Could you check a few things on this model? Use its own coordinates, in mm. A direction names the side the tool comes from. Coordinates: 2 decimals unless noted, no trailing zeros. Loops run counter-clockwise (first coordinate to the right, second up) from the corner with the lowest first, then second, coordinate; pieces in that order, holes last. Notation, with made-up numbers: (34, 30) - (91, 30) arc R14 cw to (91, 41) - close; hole circle Ø8 at (-33.75, 44). An arc over 180 degrees is marked (long way). One line per item, written item: value. Start each with the question number.
(1) If we section it at C-C on x = -20: Write out the boundary of the cut face in (y, z).
(2) If I drill on line 1 along X through (y, z) = (-30.5, 3.25); line 2 along Z through (x, y) = (-55, -6); line 3 along Y through (x, z) = (-43.5, 1.5), over which ranges is the centre line in solid material (lowest first)? Write a range as from..to.
(3) If we section it at A-A on x = -3.5: Write out the boundary of the cut face in (y, z).
(4) On a 3-axis mill with a long thin cutter (end or side, diameter ignored), from which of +Z, -Z, +X, -X, +Y, -Y can I reach the whole of each face in a straight line? I mean faces 1 (the face through (-38, 0, 0)), 2 (the face through (-61, -25, 4)), 3 (the face through (-48, 27, 3)), 4 (the face through (-48, -27, 3)), 5 (the face through (-59.972, 11.198, 1.014)). Say none if no direction works.
(5) If we section it at B-B on y = -19: Write out the boundary of the cut face in (x, z), then the cut area to 3 significant figures.
(6) I'm going to push flat-ended pins straight in: P1, Ø12, axis at x = -40.5, y = -14.5, coming from the +Z side; P2, Ø0.6, axis at y = -2.5, z = 1.5, coming from the -X side; P3, Ø2, axis at x = -21, z = 1, coming from the +Y side. Where does each tip first touch, or does it pass through?
(7) If we mould it in two halves opening along X, with no side actions, what happens to faces 6 (the face through (-55, 35, 1)), 7 (the face through (-4.75, -0.1, 0.99)), 8 (the face through (-60.028, -11.302, 1.014)), 9 (the face through (-60, 30, 4))? For each: pulls with the +X half, pulls with the -X half, needs draft (parallel to the pull), parting line crosses it, or undercut.
```python
from build123d import *

# Parameters (mm, degrees)
F1_DEPTH = 2
F0_W     = 2
F0_H     = 10
F2_DEPTH = 7
F5_DEPTH = 25


with BuildPart() as f1:
    # F0 (on Top) → F1 (new body)
    with BuildSketch(Plane.XY):
        with BuildLine():
            Line((0, 15), (-48, 15))
            Line((-48, 15), (-48, 25))
            Line((-48, 25), (-50, 25))
            Line((-50, 25), (-50, 35))
            Line((-50, 35), (-60, 35))
            Line((-60, 35), (-60, 25))
            Line((-60, 25), (-62, 25))
            Line((-62, 25), (-62, -25))
            Line((-62, -25), (-60, -25))
            Line((-60, -25), (-60, -35))
            Line((-60, -35), (-50, -35))
            Line((-50, -35), (-50, -25))
            Line((-50, -25), (-48, -25))
            Line((-48, -25), (-48, -15))
            Line((-48, -15), (0, -15))
            Line((0, -15), (0, -4.75))
            ThreePointArc((0, -4.75), (-4.75, 0), (0, 4.75))
            Line((0, 4.75), (0, 15))
        make_face()
    extrude(amount=F1_DEPTH)

    # F0 (on Top) → F2 (join)
    with BuildSketch(Plane.XY):
        with Locations((-61, 30)):
            Rectangle(F0_W, F0_H)
        with Locations((-49, 30)):
            Rectangle(F0_W, F0_H)
        with Locations((-61, -30)):
            Rectangle(F0_W, F0_H)
        with Locations((-49, -30)):
            Rectangle(F0_W, F0_H)
    extrude(amount=F2_DEPTH)

    # F4 (on face) → F5 (cut)
    with BuildSketch(Plane.XY.offset(2)):
        Polygon((-62, 15), (-62, -15), (-58, -7.5), (-58, 7.5), align=None)
    extrude(amount=-F5_DEPTH, mode=Mode.SUBTRACT)


solid = f1.part
```
Values:
1. outline: (-15, 0) - (15, 0) - (15, 2) - (-15, 2) - close
2. line 1: x = -62..-60, -50..-48
2. line 2: z = 0..2
2. line 3: y = -15..15
3. outline: (-15, 0) - (-3.21, 0) - (-3.21, 2) - (-15, 2) - close; (3.21, 0) - (15, 0) - (15, 2) - (3.21, 2) - close
4. face 1: -Z, +X, -X, +Y, -Y
4. face 2: +Z, +X, -X
4. face 3: +Z, -Z, +X, +Y
4. face 4: +Z, -Z, +X, -Y
4. face 5: +Z, -Z, -X
5. outline: (-62, 0) - (-48, 0) - (-48, 2) - (-62, 2) - close
5. area: 28.0 mm2
6. P1: stops at z = 2
6. P2: stops at x = -58
6. P3: stops at y = 15
7. face 6: needs draft
7. face 7: pulls with the +X half
7. face 8: pulls with the -X half
7. face 9: undercut
